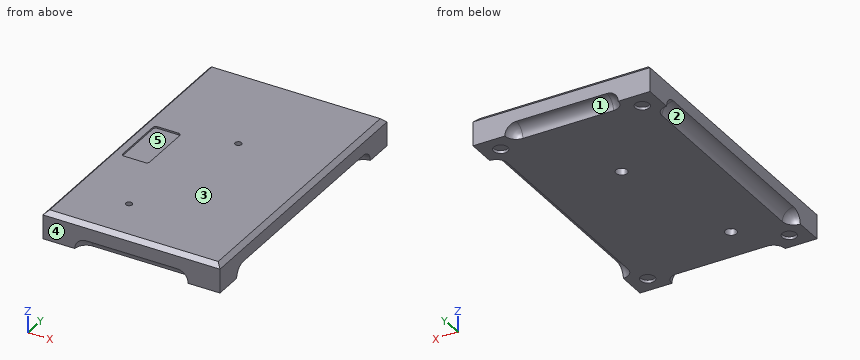
Autodesk Inventor part; units mm, degrees
ref_plane "YZ Plane" through (0, 0, 0) normal (1, 0, 0) x (0, 1, 0)
ref_plane "XZ Plane" through (0, 0, 0) normal (0, 1, 0) x (-1, 0, 0)
ref_plane "XY Plane" through (0, 0, 0) normal (0, 0, 1) x (1, 0, 0)
sketch "Skizze1" plane through (0, 0, 0) normal (0, 0, 1) x (1, 0, 0)
  line L0 (-87.5, 0) -> (87.5, 0)
  line L1 (0, -140) -> (0, 140)
  line L2 (-62.5, 100) -> (62.5, 100)
  line L3 (62.5, 100) -> (62.5, -100)
  line L4 (62.5, -100) -> (-62.5, -100)
  line L5 (-62.5, -100) -> (-62.5, 100)
  point P0 (0, 0)
  dimension "d0" = 125
  dimension "d1" = 200
extrude "Grundkörper" add sketch "Skizze1" along normal blind 20
chamfer "umlaufende Fase 3x45°" distance 3 angle 45 4 edges at (0, -100, 20) (62.5, 0, 20) (0, 100, 20) (-62.5, 0, 20)
sketch "Fräsung Rund" plane through (-62.5, -100, 0) normal (0, -1, 0) x (1, 0, 0)
  line L0 (62.5, -4) -> (62.5, 24)
  line L1 (-25, 0) -> (150, 0)
  line L2 (125, 0) -> (0, 0)
  line L3 (30.5, 8) -> (94.5, 8)
  arc A0 (102.5, 0) -> (94.5, 8) centre (94.5, 0) ccw
  arc A1 (30.5, 8) -> (22.5, 0) centre (30.5, 0) ccw
  point P0 (62.5, 0)
  dimension "d13" = 80
  dimension "d14" = 8
  dimension "d15" = 8
  dimension "d16" = 8
extrude "Querfräsung 80" cut sketch "Fräsung Rund" against normal blind 8
fillet "Rundung Querfräsung" radius 8 3 edges at (37.6569, -92, 5.6569) (-37.6569, -92, 5.6569) (0, -92, 8)
mirror "Spiegeln Querfräsung" about plane through (0, 0, 0) normal (0, 1, 0) of "Querfräsung 80", "Rundung Querfräsung"
sketch "Skizze5" plane through (62.5, -100, 0) normal (1, 0, 0) x (0, 0, -1)
  line L0 (0, -40) -> (0, 240)
  line L1 (4, 100) -> (-24, 100)
  line L2 (0, 200) -> (0, 0)
  arc A0 (-8, 28) -> (0, 20) centre (0, 28) ccw
  arc A1 (0, 180) -> (-8, 172) centre (0, 172) ccw
  line L3 (-8, 28) -> (-8, 172)
  point P0 (0, 100)
  dimension "d21" = 8
  dimension "d22" = 8
  dimension "d23" = 8
  dimension "d24" = 160
extrude "Längsfräsung 160" cut sketch "Skizze5" against normal blind 8
fillet "Rundung Längsfräsung" radius 8 3 edges at (54.5, 77.6569, 5.6569) (54.5, -77.6569, 5.6569) (54.5, 0, 8)
mirror "Spiegeln Längsfräsung" about plane through (0, 0, 0) normal (1, 0, 0) of "Längsfräsung 160", "Rundung Längsfräsung"
sketch "Skizze6" plane through (0, 0, 20) normal (0, 0, 1) x (1, 0, 0)
  line L0 (-87.5, 0) -> (87.5, 0)
  line L1 (0, -140) -> (0, 140)
  line L2 (-54.5, -20) -> (-35.5, -20)
  line L3 (-35.5, -20) -> (-35.5, 20)
  line L4 (-35.5, 20) -> (-54.5, 20)
  line L5 (-54.5, 20) -> (-54.5, -20)
  line L6 (-62.5, 100) -> (-62.5, -100)
  point P0 (0, 0)
  dimension "d28" = 19
  dimension "d29" = 40
  dimension "d34" = 8
extrude "Tasche 40x19x1,2" cut sketch "Skizze6" against normal blind 1.2
fillet "Rundung Tasche" radius 2 4 edges at (-54.5, 20, 19.4) (-54.5, -20, 19.4) (-35.5, 20, 19.4) (-35.5, -20, 19.4)
sketch "Skizze9" plane through (0, 0, 0) normal (0, 0, -1) x (-1, 0, 0)
  line L0 (-62.5, -100) -> (-40, -100)
  line L1 (0, -140) -> (0, 140)
  line L2 (87.5, 0) -> (-87.5, 0)
  line L3 (62.5, -100) -> (62.5, -80)
  line L4 (40, -100) -> (62.5, -100)
  point P0 (0, 0)
  point P1 (21.5, -66.5)
  point P2 (0, 28)
  dimension "d65" = 33.5
  dimension "d66" = 94.5
  dimension "d67" = 21.5
hole "Durchgangsbohrung Ø4,5" at (-21.5, -66.5, 0) at (0, 28, 0) direction (0, 0, 1) diameter 4.5 end through all counterbore diameter 8 counterbore depth 4.6
sketch "Skizze10" plane through (0, 0, 0) normal (0, 0, -1) x (-1, 0, 0)
  line L0 (-32, 100) -> (32, 100)
  line L1 (62.5, 72) -> (62.5, -72)
  line L2 (-87.5, 0) -> (87.5, 0)
  line L3 (0, -140) -> (0, 140)
  circle A0 centre (-50, 88) radius 5
  circle A1 centre (50, 88) radius 5
  circle A2 centre (-50, -88) radius 5
  circle A3 centre (50, -88) radius 5
  point P0 (0, 0)
  dimension "d68" = 50
  dimension "d69" = 100
  dimension "d70" = 176
  dimension "d71" = 176
  dimension "d72" = 50
  dimension "d73" = 100
  dimension "d74" = 10
  dimension "d75" = 10
  dimension "d76" = 10
  dimension "d77" = 10
extrude "Extrusion5" cut sketch "Skizze10" against normal blind 2
properties part number "Grundplatte"
Can you work these out from the model? Positions are in its coordinate system, mm. Face numbers are marked on the shaded views. A direction names the side the tool comes from. Round coordinates to 2 decimals unless told otherwise and drop trailing zeros. Loops run counter-clockwise (first coordinate to the right, second up) from the corner with the lowest first, then second, coordinate; pieces in that order, holes last. Notation, with made-up numbers: (79.25, 54) - (96.25, 54) arc R34 ccw to (96.25, 85) - close; hole circle Ø6 at (25, 25.25). An arc over 180 degrees is marked (long way). Answer in a Markdown table with one row per item. Add a question column.
Q1. We'd pull the mould along Y, two halves only. Please class the marked faces 1, 2 and 3: pulls with the +Y half, pulls with the -Y half, needs draft (parallel to the pull), parting line crosses it, or undercut.
Q2. I need wall thicknesses on L1, parallel to Y at x = 50, z = 1.2; L2, parallel to Y at x = 0, z = 13.75; L3, parallel to X at y = -66.5, z = 16.25. Which ranges of each line are inside material? Lowest first, please.
Q3. For pin 1 Ø1.5 at (x, z) = (-22, 18) entering from +Y; pin 2 Ø1 at (y, z) = (4, 19.5) entering from -X; pin 3 Ø3.5 at (x, y) = (-21.5, -66.5) entering from +Z; pin 4 Ø5 at (x, y) = (0, 28) entering from -Z, each with a flat end and sliding along its axis, tell me the tip position at first contact or that it passes through.
Q4. I want a section at D-D on x = -50. List the corners of the cut face in (y, z) for me.
Q5. Which directions (+Z, -Z, +X, -X, +Y, -Y) give clear straight access to the entire face, cutting with the end or side of a thin tool? Please do the marked faces 4 and 5.
A:
| question | item | result |
|---|---|---|
| 1 | face 1 | pulls with the +Y half |
| 1 | face 2 | undercut |
| 1 | face 3 | needs draft |
| 2 | L1 | -100 to -93, -83 to 83, 93 to 100 |
| 2 | L2 | -100 to 25.75, 30.25 to 100 |
| 2 | L3 | -62.5 to -23.75, -19.25 to 62.5 |
| 3 | pin 1 | y = 99.75 |
| 3 | pin 2 | x = -60.5 |
| 3 | pin 3 | through |
| 3 | pin 4 | z = 4.6 |
| 4 | outline | (-100, 0) - (-93, 0) - (-93, 2) - (-83, 2) - (-83, 0) - (83, 0) - (83, 2) - (93, 2) - (93, 0) - (100, 0) - (100, 17) - (97, 20) - (20, 20) - (20, 18.8) - (-20, 18.8) - (-20, 20) - (-97, 20) - (-100, 17) - close |
| 5 | face 4 | +Z, -Z, +X, -X, -Y |
| 5 | face 5 | +Z |
